For this review, take the finished solid that the model builds, in its own axes (mm). A direction names the side the tool comes from. Give positions to 0.01 mm unless a question says otherwise; leave off trailing zeros. Write each loop counter-clockwise with the first axis right and the second up, starting at its lowest first coordinate (ties: lowest second). Pieces come first, ordered by that corner, then holes. Notation, with made-up numbers: M 50.25,-25.75 L 107.25,-25.75 A16 cw 107.25,-5.75 Z; hole C 4,-38 d11. An arc over 180 degrees is marked long. Write item = value, one per line.
```python
from build123d import *

# Parameters (mm, degrees)
SKETCH1_W                                    = 162
SKETCH1_H                                    = 100
SKETCH1_W_2                                  = 50
SKETCH1_H_2                                  = 4
SKETCH1_W_3                                  = 4
SKETCH1_H_3                                  = 50
BOSS_EXTRUDE2_DEPTH                          = 4
CUT_EXTRUDE1_REACH                           = 102.782
SKETCH2_R                                    = 12
CSK_FOR_M4_COUNTERSUNK_FLAT_HEAD_SCR_2_COUNT = 2
CSK_FOR_M4_COUNTERSUNK_FLAT_HEAD_SCR_2_PITCH = 142
CSK_FOR_M4_COUNTERSUNK_FLAT_HEAD_SCR_3_COUNT = 2
CSK_FOR_M4_COUNTERSUNK_FLAT_HEAD_SCR_3_PITCH = 162.984661855
CSK_FOR_M4_COUNTERSUNK_FLAT_HEAD_SCR_4_COUNT = 2
CSK_FOR_M4_COUNTERSUNK_FLAT_HEAD_SCR_4_PITCH = 80
F_3_0MM_DOWEL_HOLE1_D                        = 3


with BuildPart() as part:
    # Sketch1 → Boss-Extrude2 (new body)
    with BuildSketch(Plane.XY):
        Rectangle(SKETCH1_W, SKETCH1_H)
        with Locations((0, 52)):
            Rectangle(SKETCH1_W_2, SKETCH1_H_2)
        with Locations((83, 0)):
            Rectangle(SKETCH1_W_3, SKETCH1_H_3)
        with Locations((-83, 0)):
            Rectangle(SKETCH1_W_3, SKETCH1_H_3)
        with Locations((0, -52)):
            Rectangle(SKETCH1_W_2, SKETCH1_H_2)
    extrude(amount=BOSS_EXTRUDE2_DEPTH)

    # Sketch2 → Cut-Extrude1 (cut, up to next)
    with BuildSketch(Plane.XY.offset(4), mode=Mode.PRIVATE) as cut_extrude1_sk1:
        with Locations((-40, 0)):
            Circle(SKETCH2_R)
    cut_extrude1_tool1 = extrude(cut_extrude1_sk1.sketch, amount=-CUT_EXTRUDE1_REACH, mode=Mode.PRIVATE) & part.part
    # Sketch2 → Cut-Extrude1 (cut, up to next)
    with BuildSketch(Plane.XY.offset(4), mode=Mode.PRIVATE) as cut_extrude1_sk2:
        with Locations((20, 0)):
            Circle(SKETCH2_R)
    cut_extrude1_tool2 = extrude(cut_extrude1_sk2.sketch, amount=-CUT_EXTRUDE1_REACH, mode=Mode.PRIVATE) & part.part
    # Sketch2 → Cut-Extrude1 (cut, up to next)
    with BuildSketch(Plane.XY.offset(4), mode=Mode.PRIVATE) as cut_extrude1_sk3:
        with Locations((50, 0)):
            Circle(SKETCH2_R)
    cut_extrude1_tool3 = extrude(cut_extrude1_sk3.sketch, amount=-CUT_EXTRUDE1_REACH, mode=Mode.PRIVATE) & part.part
    add(cut_extrude1_tool1.solids().sort_by_distance((-40, 0, 4))[0], mode=Mode.SUBTRACT)
    add(cut_extrude1_tool2.solids().sort_by_distance((20, 0, 4))[0], mode=Mode.SUBTRACT)
    add(cut_extrude1_tool3.solids().sort_by_distance((50, 0, 4))[0], mode=Mode.SUBTRACT)

    # Sketch4 → CSK for M4 Countersunk Flat Head Screw1 (revolve, cut)
    with BuildSketch(Plane(origin=(-71, 40, 4), x_dir=(0, -1, 0), z_dir=(1, 0, 0))):
        Polygon((0, 0), (0, 4), (2.25, 4), (2.25, 2.45), (4.7, 0), align=None)
    csk_for_m4_countersunk_flat_head_screw1 = revolve(axis=Axis((-71, 40, 10.35), (0, 0, -1)), mode=Mode.SUBTRACT)

    # CSK for M4 Countersunk Flat Head Scr 2: CSK for M4 Countersunk Flat Head Screw1 ×2
    with Locations(*[(i * CSK_FOR_M4_COUNTERSUNK_FLAT_HEAD_SCR_2_PITCH, 0, 0) for i in range(1, CSK_FOR_M4_COUNTERSUNK_FLAT_HEAD_SCR_2_COUNT)]):
        add(csk_for_m4_countersunk_flat_head_screw1, mode=Mode.SUBTRACT)

    # CSK for M4 Countersunk Flat Head Scr 3: CSK for M4 Countersunk Flat Head Screw1 ×2
    with Locations(*[Vector(0.8712476277448776, -0.49084373394077596, 0) * (i * CSK_FOR_M4_COUNTERSUNK_FLAT_HEAD_SCR_3_PITCH) for i in range(1, CSK_FOR_M4_COUNTERSUNK_FLAT_HEAD_SCR_3_COUNT)]):
        add(csk_for_m4_countersunk_flat_head_screw1, mode=Mode.SUBTRACT)

    # CSK for M4 Countersunk Flat Head Scr 4: CSK for M4 Countersunk Flat Head Screw1 ×2
    with Locations(*[(0, -i * CSK_FOR_M4_COUNTERSUNK_FLAT_HEAD_SCR_4_PITCH, 0) for i in range(1, CSK_FOR_M4_COUNTERSUNK_FLAT_HEAD_SCR_4_COUNT)]):
        add(csk_for_m4_countersunk_flat_head_screw1, mode=Mode.SUBTRACT)

    # Ø3.0mm Dowel Hole1 (through all)
    with Locations(Plane(origin=(-49.5, 12, 4), x_dir=(1, 0, 0), z_dir=(0, 0, 1))):
        with Locations((0, 0), (19, -24), (60, 0), (79, -24), (90, 0), (109, -24)):
            Hole(F_3_0MM_DOWEL_HOLE1_D / 2)


solid = part.part
```
1. For line 1 along X through (y, z) = (-8, 1.2); line 2 along X through (y, z) = (-10, 3); line 3 along Y through (x, z) = (-54.5, 1.5), list the stretches that pass through material, from the lowest coordinate up. Write a range as from..to.
Responses:
line_1 = -85..-48.94, -31.06..11.06, 28.94..41.06, 58.94..85
line_2 = -85..-46.63, -33.37..13.37, 26.63..43.37, 56.63..85
line_3 = -50..50
2. Insertion check: P1, Ø1.2, axis at y = 43.5, z = 2.5, coming from the -X side; P2, Ø2, axis at y = -51.5, z = 1.5, coming from the +X side; P3, Ø1.8, axis at x = -49.5, y = 12, coming from the -Z side; P4, Ø1, axis at x = -62.5, z = 1.5, coming from the +Y side. Each pin has a flat end and moves straight along its axis. Give the tip position at first contact, or say it passes through.
Responses:
P1 = -81
P2 = 25
P3 = through
P4 = 50
3. We need section C-C, the plane y = 0. Write out the cut boundary in (x, z).
Responses:
outline = M -85,0 L -52,0 L -52,4 L -85,4 Z; M -28,0 L 8,0 L 8,4 L -28,4 Z; M 32,0 L 38,0 L 38,4 L 32,4 Z; M 62,0 L 85,0 L 85,4 L 62,4 Z
4. Machinability: for faces 1 (the face through (-49.523, -7.302, 2.028)), 2 (the face through (-81, 37, 2)), 3 (the face through (-83, -25, 2)), 4 (the face through (81, -38, 2)), which of the approach directions +Z, -Z, +X, -X, +Y, -Y give a long, thin tool a straight path to every point of the face, cutting with its end or side? Answer none if there is none.
Responses:
face_1 = +Z, -Z
face_2 = +Z, -Z, -X, +Y
face_3 = +Z, -Z, -X, -Y
face_4 = +Z, -Z, +X, -Y
5. We need section B-B, the plane x = 50. Write out the cut boundary in (y, z).
Responses:
outline = M -50,0 L -12,0 L -12,4 L -50,4 Z; M 12,0 L 50,0 L 50,4 L 12,4 Z
6. The part is to be moulded in two halves that separate along X. For faces 5 (the face through (69.38, -38.23, 1.7)), 6 (the face through (81, 37, 2)), 7 (the face through (83, 25, 2)), say which applies: +X half, -X half, draft (parallel to the pull), parting line (faces both ways), or undercut.
Responses:
face_5 = undercut
face_6 = +X half
face_7 = draft
7. We need section A-A, the plane y = -40. Write out the cut boundary in (x, z).
Responses:
outline = M -81,0 L -73.25,0 L -73.25,1.55 L -75.7,4 L -81,4 Z; M -68.75,0 L 68.75,0 L 68.75,1.55 L 66.3,4 L -66.3,4 L -68.75,1.55 Z; M 73.25,0 L 81,0 L 81,4 L 75.7,4 L 73.25,1.55 Z
8. We need section D-D, the plane z = 0.65. Count the separate pieces of the cut face and the enclosed holes in it, then the cut area to 3 significant figures.
Responses:
separate_pieces = 1
enclosed_holes = 13
area = 15,500 mm2
